The model under review builds one solid part; all positions refer to its coordinate system, in mm. Round coordinates to 2 decimals unless told otherwise and drop trailing zeros. Order: outer loops, then holes, each group sorted by start corner. A loop starts at its lowest first (then second) coordinate and runs counter-clockwise, first axis right, second up.
1) Consider section B-B (z = 6.75). Give the number of separate pieces and of enclosed holes in the cut face, then the cut area to 3 significant figures.
2) Mouldability with a two-part tool opening along Y and no side actions: class faces 1 (the face through (147, 20, 5)), 2 (the face through (6, 10, 5)), 3 (the face through (146, 10, 0)) as pulls with the +Y half, pulls with the -Y half, needs draft (parallel to the pull), parting line crosses it, or undercut.
3) Consider section A-A (x = 277). Give the boundary of the cut face in (y, z).
4) Clearance check with flat-ended pins moving along their axes: P1, Ø1, axis at y = 13.5, z = 7.5, coming from the -X side; P2, Ø1, axis at y = 6.5, z = 4.5, coming from the +X side. State where each tip first meets the part, or that it passes through.
5) To check wall thickness, follow L1, parallel to Y at x = 103.5, z = 5.5; L2, parallel to Y at x = 10, z = 3.75; L3, parallel to X at y = 7.75, z = 4. State the ranges of each line that lie inside material, in increasing order.
6) Consider section C-C (y = 3.25). Give the boundary of the cut face in (x, z).
from build123d import *

# Parameters (mm, degrees)
ESQUISSE1_W        = 297
ESQUISSE1_H        = 20
ESQUISSE1_R        = 4
ESQUISSE1_R_2      = 2.5
ESQUISSE1_R_3      = 2
BOSS_EXTRU_1_DEPTH = 10
CONG_1_R           = 10


with BuildPart() as part:
    # Esquisse1 → Boss.-Extru.1 (new body)
    with BuildSketch(Plane.XY):
        with Locations((148.5, 10)):
            Rectangle(ESQUISSE1_W, ESQUISSE1_H)
        with Locations((10, 10)):
            Circle(ESQUISSE1_R, mode=Mode.SUBTRACT)
        with Locations((54, 10)):
            Circle(ESQUISSE1_R, mode=Mode.SUBTRACT)
        with Locations((277, 10)):
            Circle(ESQUISSE1_R_2, mode=Mode.SUBTRACT)
        with Locations((287, 10)):
            Circle(ESQUISSE1_R_2, mode=Mode.SUBTRACT)
        with Locations((103.5, 10)):
            Circle(ESQUISSE1_R_3, mode=Mode.SUBTRACT)
        with Locations((193.5, 10)):
            Circle(ESQUISSE1_R_3, mode=Mode.SUBTRACT)
    extrude(amount=BOSS_EXTRU_1_DEPTH)

    # Congé1
    cong_1_edges = [part.edges().sort_by_distance(p)[0] for p in [
        (0, 0, 5),
        (0, 20, 5),
        (297, 0, 5),
        (297, 20, 5),
    ]]
    fillet(cong_1_edges, radius=CONG_1_R - 0.0001)  # a hair under: the kernel refuses the full size


solid = part.part
Answer below:
1. separate pieces: 1
1. enclosed holes: 6
1. area: 5,690 mm2
2. face 1: pulls with the +Y half
2. face 2: undercut
2. face 3: needs draft
3. outline: (0, 0) - (7.5, 0) - (7.5, 10) - (0, 10) - close; (12.5, 0) - (20, 0) - (20, 10) - (12.5, 10) - close
4. P1: stops at x = 0.46
4. P2: stops at x = 296.54
5. L1: y = 0 to 8, 12 to 20
5. L2: y = 0 to 6, 14 to 20
5. L3: x = 0.26 to 6.69, 13.31 to 50.69, 57.31 to 275.91, 278.09 to 285.91, 288.09 to 296.74
6. outline: (2.62, 0) - (294.38, 0) - (294.38, 10) - (2.62, 10) - close
